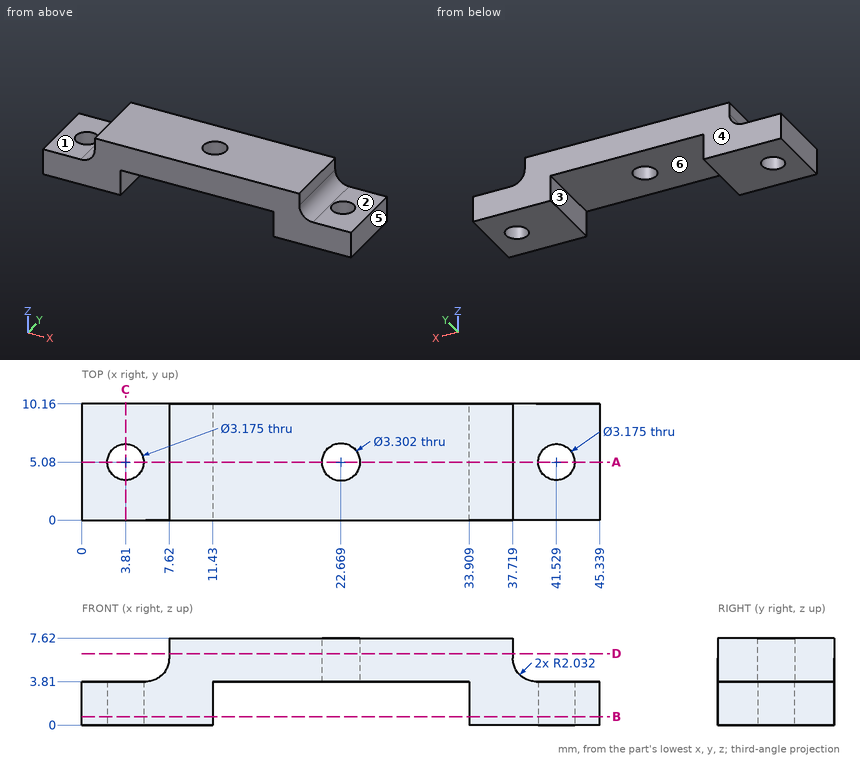
Design review of the part shown in the three views and the two pictorial views. Dimensions are in mm from the part's minimum x, y and z. A direction names the side the tool comes from. Coordinates: 2 decimals unless noted, no trailing zeros. Write each loop counter-clockwise with the first axis right and the second up, starting at its lowest first coordinate (ties: lowest second). Pieces come first, ordered by that corner, then holes. Notation, with made-up numbers: (13.5, 37) - (54.5, 37) arc R22 cw to (54.5, 54) - close; hole circle Ø7 at (69.25, 36.25). An arc over 180 degrees is marked (long way). Write item = value, one per line.
(1) Mouldability with a two-part tool opening along X and no side actions: class the marked faces 4, 5 and 6 as pulls with the +X half, pulls with the -X half, needs draft (parallel to the pull), parting line crosses it, or undercut.
Result sheet:
face_4 = needs draft
face_5 = pulls with the +X half
face_6 = undercut
(2) Consider section C-C, the plane x = 3.81. Give the boundary of the cut face in (y, z).
Result sheet:
outline = (0, 0) - (3.49, 0) - (3.49, 3.81) - (0, 3.81) - close; (6.67, 0) - (10.16, 0) - (10.16, 3.81) - (6.67, 3.81) - close
(3) Consider section A-A, the plane y = 5.08. State how many separate pieces and enclosed holes the cut face has, then the cut area to 3 significant figures.
Result sheet:
separate_pieces = 4
enclosed_holes = 0
area = 167 mm^2
(4) For line 1 (X direction, y = 5.08, z = 1.75); line 2 (X direction, y = 5.25, z = 2.75); line 3 (Z direction, x = 4, y = 8), list the stretches that pass through material, from the lowest coordinate up. Write a range as [from, to].
Result sheet:
line_1 = [0, 2.22], [5.4, 11.43], [33.91, 39.94], [43.12, 45.34]
line_2 = [0, 2.23], [5.39, 11.43], [33.91, 39.95], [43.11, 45.34]
line_3 = [0, 3.81]
(5) Consider section B-B, the plane z = 0.75. Give the boundary of the cut face in (x, y) (1 decimal).
Result sheet:
outline = (0, 0) - (11.4, 0) - (11.4, 10.2) - (0, 10.2) - close; (33.9, 0) - (45.3, 0) - (45.3, 10.2) - (33.9, 10.2) - close; hole circle Ø3.2 at (3.8, 5.1); hole circle Ø3.2 at (41.5, 5.1)
(6) For P1, Ø4, axis at x = 22.67, y = 5.08, coming from the +Z side; P2, Ø3.5, axis at x = 41.529, y = 5.08, coming from the +Z side; P3, Ø1.4, axis at y = 3.5, z = 6.5, coming from the +X side; P4, Ø1.4, axis at y = 3, z = 7, coming from the -X side, all flat-tipped, find the tip position at first contact; note any pin that passes through.
Result sheet:
P1 = 7.62
P2 = 3.81
P3 = 37.72
P4 = 7.62
(7) Consider section D-D, the plane z = 6.25. Give the boundary of the cut face in (x, y).
Result sheet:
outline = (7.62, 0) - (37.72, 0) - (37.72, 10.16) - (7.62, 10.16) - close; hole circle Ø3.3 at (22.67, 5.08)
(8) Machinability: for the marked faces 1, 2 and 3, which of the approach directions +Z, -Z, +X, -X, +Y, -Y give a long, thin tool a straight path to every point of the face, cutting with its end or side? Answer none if there is none.
Result sheet:
face_1 = +Z, -X, +Y, -Y
face_2 = +Z, +X, +Y, -Y
face_3 = -Z, +Y, -Y
